Here's how the part is built. I have some questions about the finished solid (model axes, mm). A direction names the side the tool comes from. Round coordinates to 2 decimals unless told otherwise and drop trailing zeros. Write each loop counter-clockwise with the first axis right and the second up, starting at its lowest first coordinate (ties: lowest second). Pieces come first, ordered by that corner, then holes. Notation, with made-up numbers: (75, 10.25) -> (134, 10.25) arc R29 cw to (134, 46.25) -> close; hole circle Ø8 at (31.25, 26.25). An arc over 180 degrees is marked (long way). Put each result on its own line as item: value. Start each with the question number.
1) Will these pins go through, and if not, where does the flat tip stop? P1, Ø4, axis at x = -2.5, z = 11, coming from the +Y side; P2, Ø7, axis at x = 0, z = 13, coming from the -Y side; P3, Ø8, axis at y = 7.5, z = 9.5, coming from the +X side; P4, Ø2.5, axis at x = 0, y = 8.5, coming from the -Z side.
2) I want a section at B-B, the plane y = 8.5. List the corners of the cut face in (x, z) for me.
3) We'd pull the mould along X, two halves only. Please class faces 1 (the cylindrical face through (0.65, 0.06, 15.05)), 2 (the cylindrical face through (8.699, -11.715, 20.972)), 3 (the flat face through (-6.5, 0.1, 9)), 4 (the flat face through (-2, -8, 19)): released by +X, released by -X, zero draft, split by the parting line, or undercut.
4) Which directions (+Z, -Z, +X, -X, +Y, -Y) give clear straight access to the entire face, cutting with the end or side of a thin tool? Please do faces 5 (the cylindrical face through (8.699, -4.715, 14.81)), 6 (the flat face through (3.4, 5, 12.7)), 7 (the flat face through (6.5, 0.1, 9)), 8 (the cylindrical face through (-8.715, 4.699, 14.81)), 9 (the cylindrical face through (0.249, 7.377, 21.479)).
5) If I drill on line 1 along Y through (x, z) = (0, 21.4); line 2 along Z through (x, y) = (5.75, 6.5); line 3 along X through (y, z) = (-9.5, 19.75), over which ranges is the centre line in solid material (lowest first)? Write a range as [from, to].
6) I want a section at C-C, the plane x = 0. List the corners of the cut face in (y, z) for me, then the cut area to 3 significant figures.
7) I want a section at A-A, the plane z = 13. List the corners of the cut face in (x, y) for me, then the cut area to 3 significant figures.
8) I want a section at D-D, the plane y = -1.25. List the corners of the cut face in (x, z) for me.
from build123d import *

# Parameters (mm, degrees)
SKETCH_1_W             = 18
SKETCH_1_H             = 10
EXTRUDE_1_DEPTH        = 23
SKETCH_3_R             = 2.15
CUT_EXTRUDE_1_DEPTH    = 23
FILLET_1_R             = 1
SKETCH_4_W             = 18
SKETCH_4_H             = 6.5
CUT_EXTRUDE_2_DEPTH    = 23
SKETCH_5_W             = 18
SKETCH_5_H             = 12
EXTRUDE_2_DEPTH        = 4
SKETCH_6_R             = 1.15
CUT_EXTRUDE_3_DEPTH    = 4
FILLET_2_R             = 1
CHAMFER_1_SIZE         = 1
FILLET_2_OF_MIRROR_1_R = 1
CHAMFER_2_SIZE         = 0.5
CUT_EXTRUDE_4_DEPTH    = 10


with BuildPart() as part:
    # 草图1 → 凸台-拉伸1 (new body)
    with BuildSketch(Plane.XY):
        Rectangle(SKETCH_1_W, SKETCH_1_H)
    extrude(amount=EXTRUDE_1_DEPTH)

    # 草图3 → 切除-拉伸1 (cut)
    with BuildSketch(Plane(origin=(0, 5, 0), x_dir=(1, 0, 0), z_dir=(0, 1, 0))):
        with Locations(Location((0, -13, 0), (0, 0, 270))):
            Circle(SKETCH_3_R)
    extrude(amount=-CUT_EXTRUDE_1_DEPTH, mode=Mode.SUBTRACT)

    # 圆角1
    fillet_1_edges = [part.edges().sort_by_distance(p)[0] for p in [
        (9, -5, 11.5),
        (-9, -5, 11.5),
        (-9, 5, 11.5),
        (9, 5, 11.5),
    ]]
    fillet(fillet_1_edges, radius=FILLET_1_R)

    # 草图4 → 切除-拉伸2 (cut)
    with BuildSketch(Plane(origin=(0, 5, 0), x_dir=(1, 0, 0), z_dir=(0, 1, 0))):
        with Locations((0, -3.25)):
            Rectangle(SKETCH_4_W, SKETCH_4_H)
    extrude(amount=-CUT_EXTRUDE_2_DEPTH, mode=Mode.SUBTRACT)

    # 草图5 → 凸台-拉伸2 (add)
    with BuildSketch(Plane.XY.offset(23)):
        with Locations((0, 6)):
            Rectangle(SKETCH_5_W, SKETCH_5_H)
    extrude_2 = extrude(amount=-EXTRUDE_2_DEPTH)

    # 草图6 → 切除-拉伸3 (cut)
    with BuildSketch(Plane(origin=(0, 0, 19), x_dir=(-1, 0, 0), z_dir=(0, 0, -1))):
        with Locations((0, 8.5)):
            Circle(SKETCH_6_R)
    cut_extrude_3 = extrude(amount=-CUT_EXTRUDE_3_DEPTH, mode=Mode.SUBTRACT)

    # 圆角2
    fillet_2_edges = [part.edges().sort_by_distance(p)[0] for p in [
        (9, 12, 21),
        (-9, 12, 21),
    ]]
    fillet(fillet_2_edges, radius=FILLET_2_R)

    # 倒角1
    chamfer_1_edges = [part.edges().sort_by_distance(p)[0] for p in [
        (1.15, 8.5, 19),
        (0, -5, 10.85),
        (0, 5, 10.85),
    ]]
    chamfer(chamfer_1_edges, length=CHAMFER_1_SIZE)

    # 镜向1: 凸台-拉伸2, 切除-拉伸3 across plane
    add(extrude_2.mirror(Plane.ZX))
    add(cut_extrude_3.mirror(Plane.ZX), mode=Mode.SUBTRACT)

    # 圆角2 of 镜向1
    fillet_2_of_mirror_1_edges = [part.edges().sort_by_distance(p)[0] for p in [
        (9, -12, 21),
        (-9, -12, 21),
    ]]
    fillet(fillet_2_of_mirror_1_edges, radius=FILLET_2_OF_MIRROR_1_R)

    # 倒角2
    chamfer_2_edges = [part.edges().sort_by_distance(p)[0] for p in [
        (1.15, -8.5, 19),
    ]]
    chamfer(chamfer_2_edges, length=CHAMFER_2_SIZE)

    # 草图7 → 切除-拉伸4 (cut)
    with BuildSketch(Plane(origin=(0, 5, 0), x_dir=(1, 0, 0), z_dir=(0, 1, 0))):
        Polygon((-9, -11.5), (-4, -6.5), (-9, -6.5), align=None)
        Polygon((9, -11.5), (4, -6.5), (9, -6.5), align=None)
    extrude(amount=-CUT_EXTRUDE_4_DEPTH, mode=Mode.SUBTRACT)


solid = part.part
Findings:
1. P1: stops at y = 5
1. P2: stops at y = -5
1. P3: stops at x = 9
1. P4: stops at z = 19.9
2. outline: (-9, 19) -> (-2.15, 19) -> (-1.15, 20) -> (-1.15, 23) -> (-9, 23) -> close; (1.15, 20) -> (2.15, 19) -> (9, 19) -> (9, 23) -> (1.15, 23) -> close
3. face 1: undercut
3. face 2: released by +X
3. face 3: released by -X
3. face 4: zero draft
4. face 5: -Z, +X, -Y
4. face 6: -Z, +X, -X, +Y
4. face 7: -Z, +X, +Y, -Y
4. face 8: -Z, -X, +Y
4. face 9: +Z, -Z
5. line 1: y = [-12, -9.65], [-7.35, 7.35], [9.65, 12]
5. line 2: z = [19, 23]
5. line 3: x = [-9, -0.57], [0.57, 9]
6. outline: (-12, 19) -> (-10.15, 19) -> (-9.65, 19.5) -> (-9.65, 23) -> (-12, 23) -> close; (-7.35, 19.5) -> (-6.85, 19) -> (-5, 19) -> (-5, 16.15) -> (-4, 15.15) -> (4, 15.15) -> (5, 16.15) -> (5, 19) -> (6.35, 19) -> (7.35, 20) -> (7.35, 23) -> (-7.35, 23) -> close; (-5, 6.5) -> (5, 6.5) -> (5, 9.85) -> (4, 10.85) -> (-4, 10.85) -> (-5, 9.85) -> close; (9.65, 20) -> (10.65, 19) -> (12, 19) -> (12, 23) -> (9.65, 23) -> close
6. area: 156 mm2
7. outline: (-9, -4) arc R1 ccw to (-8, -5) -> (-3.15, -5) -> (-2.15, -4) -> (-2.15, 4) -> (-3.15, 5) -> (-8, 5) arc R1 ccw to (-9, 4) -> close; (2.15, -4) -> (3.15, -5) -> (8, -5) arc R1 ccw to (9, -4) -> (9, 4) arc R1 ccw to (8, 5) -> (3.15, 5) -> (2.15, 4) -> close
7. area: 134 mm2
8. outline: (-9, 11.5) -> (-4, 6.5) -> (4, 6.5) -> (9, 11.5) -> (9, 23) -> (-9, 23) -> close; hole circle Ø4.3 at (0, 13)
